Geometry check sheet. Reference: the model listing, model coordinates, mm. A direction names the side the tool comes from. Round coordinates to 2 decimals unless told otherwise and drop trailing zeros. Order: outer loops, then holes, each group sorted by start corner. A loop starts at its lowest first (then second) coordinate and runs counter-clockwise, first axis right, second up. Notation, with made-up numbers: (25, 58.5) - (38, 58.5) arc R32 cw to (38, 86.5) - close; hole circle Ø4 at (39, 10). An arc over 180 degrees is marked (long way). Use a Markdown table: item, result. Add a question column.
(1) Section check C-C on z = 1.2. Record the boundary of the cut face in (x, y), then the cut area to 3 significant figures.
(2) Thickness scan on line 1 along Y through (x, z) = (-0.1, 2.3); line 2 along X through (y, z) = (0.7, 0.1); line 3 along Y through (x, z) = (0, 1.75). Record the ranges inside material, lowest first. Write a range as [from, to].
(3) Access from +Z, -Z, +X, -X, +Y, -Y to the whole of each face (thin tool, end or side, straight path). Record for faces 3 (the face through (-2, 1, 0.254)), 4 (the face through (1.43, 0.45, 1.24)).
(4) Mould release check, pull along X, two halves, no side actions. Record for faces 1 (the face through (0, 3, 1)), 2 (the face through (2, 1, 2.248)): released by +X, released by -X, zero draft, split by the parting line, or undercut.
(5) Gauge pin test, flat end, axial feed: P1, Ø1, axis at y = -1.5, z = 2, coming from the -X side. Record the tip position at first contact, or that the pin passes through.
```python
from build123d import *

# Parameters (mm, degrees)
SKETCH1_R          = 2.99974
SKETCH1_R_2        = 1.4986
EXTRUDE1_DEPTH     = 2.5019
FILLET1_R          = 0.127
SKETCH2_R          = 2.625078694
SKETCH2_R_2        = 1.99585199
CUT_EXTRUDE1_DEPTH = 0.254
SKETCH3_R          = 2.62509
SKETCH3_R_2        = 1.9939
CUT_EXTRUDE2_DEPTH = 0.254


with BuildPart() as part:
    # Sketch1 → Extrude1 (new body)
    with BuildSketch(Plane.XY):
        Circle(SKETCH1_R)
        Circle(SKETCH1_R_2, mode=Mode.SUBTRACT)
    extrude(amount=EXTRUDE1_DEPTH)

    # Fillet1
    fillet1_edges = [part.edges().sort_by_distance(p)[0] for p in [
        (-2.99974, 0, 0),
        (-2.99974, 0, 2.5019),
        (-1.4986, 0, 0),
        (-1.4986, 0, 2.5019),
    ]]
    fillet(fillet1_edges, radius=FILLET1_R)

    # Sketch2 → Cut-Extrude1 (cut)
    with BuildSketch(Plane.XY.offset(2.5019)):
        Circle(SKETCH2_R)
        Circle(SKETCH2_R_2, mode=Mode.SUBTRACT)
    extrude(amount=-CUT_EXTRUDE1_DEPTH, mode=Mode.SUBTRACT)

    # Sketch3 → Cut-Extrude2 (cut)
    with BuildSketch(Plane(origin=(0, 0, 0), x_dir=(-1, 0, 0), z_dir=(0, 0, -1))):
        Circle(SKETCH3_R)
        Circle(SKETCH3_R_2, mode=Mode.SUBTRACT)
    extrude(amount=-CUT_EXTRUDE2_DEPTH, mode=Mode.SUBTRACT)


solid = part.part
```
Check sheet entries:
| question | item | result |
|---|---|---|
| 1 | outline | circle Ø6 at (0, 0); hole circle Ø3 at (0, 0) |
| 1 | area | 21.2 mm2 |
| 2 | line 1 | y = [-3, -2.62], [-1.99, -1.5], [1.5, 1.99], [2.62, 3] |
| 2 | line 2 | x = [-2.91, -2.53], [-1.87, -1.33], [1.33, 1.87], [2.53, 2.91] |
| 2 | line 3 | y = [-3, -1.5], [1.5, 3] |
| 3 | face 3 | -Z |
| 3 | face 4 | +Z, -Z |
| 4 | face 1 | split by the parting line |
| 4 | face 2 | undercut |
| 5 | P1 | stops at x = -2.83 |
